Read the model definition and answer for the solid it produces. Units are mm, in the model's axes. A direction names the side the tool comes from. Coordinates: 2 decimals unless noted, no trailing zeros. Order: outer loops, then holes, each group sorted by start corner. A loop starts at its lowest first (then second) coordinate and runs counter-clockwise, first axis right, second up. Notation, with made-up numbers: (15, -25) -> (58, -25) arc R29 ccw to (58, 6) -> close; hole circle Ø5 at (79, 64.25). An arc over 180 degrees is marked (long way). Answer as a JSON object with one key per item and string values. Group by question number.
1) Section C-C on z = 34.5 is taken. Determine the outline of the cut face in (x, y) (3 decimals), and give its area (3 significant figures).
2) Section D-D on y = -20 is taken. Determine the outline of the cut face in (x, z) (3 decimals), and give its area (3 significant figures).
3) Section A-A on y = 0 is taken. Determine the outline of the cut face in (x, z) (3 decimals).
4) A tool of negligible diameter and unlimited length cuts with its end or side. For faces 1 (the cylindrical face through (30.18, 0.39, 66.19)), 2 (the flat face through (28.575, 0, 28)), from which of +Z, -Z, +X, -X, +Y, -Y can it reach the whole face along a straight path? Write none if from no direction.
5) Consider L1, parallel to Z at x = 30.8, y = 0; L2, parallel to X at y = -22, z = 9.5 (3 decimals); L3, parallel to Z at x = 25.5, y = -27 (3 decimals). Determine where each line is inside the solid, lowest interval first.
6) Determine the mould class of faces 3 (the cylindrical face through (30.18, -0.83, 59.79)), 4 (the flat face through (-31.75, 0, 25)), 5 (the flat face through (-28.575, 0, 28)), 6 (the flat face through (0, 0, 3.175)) for opening direction X: released by +X, released by -X, zero draft, split by the parting line, or undercut.
7) Given pin 1 (3 mm diameter, centred on x = -1, y = 7.5, fed in from -Z); pin 2 (8 mm diameter, centred on x = 24, z = 44.5, fed in from -Y); pin 3 (1 mm diameter, centred on x = -23.5, y = -5.5, fed in from +Z) (3 decimals), each flat-ended and moving along its own axis, determine where each tip first touches the part or whether it passes through.
8) Section B-B on z = 56 is taken. Determine the outline of the cut face in (x, y) (3 decimals).
from build123d import *

# Parameters (mm, degrees)
F0_W     = 31.75
F0_H     = 63.5
F1_DEPTH = 3.175
F2_R     = 6.35
F3_DEPTH = 3.175


with BuildPart() as f1:
    # F0 (on Top) → F1 (new body)
    with BuildSketch(Plane.XY):
        with Locations((15.875, 0)):
            Rectangle(F0_W, F0_H)
    extrude(amount=F1_DEPTH)

    # F2 (on face) → F3 (join)
    with BuildSketch(Plane.YZ.offset(31.75)):
        Polygon((-10.280992, 46.040436), (-30.269473, 3.175), (30.269473, 3.175), (10.280992, 46.040436), align=None)
        with BuildLine():
            ThreePointArc((10.280992, 46.040436), (0, 66.196386), (-10.280992, 46.040436))
            Line((-10.280992, 46.040436), (10.280992, 46.040436))
        make_face()
        with Locations((0, 53.496386)):
            Circle(F2_R, mode=Mode.SUBTRACT)
    extrude(amount=-F3_DEPTH)

    # F4: F1 across plane


with BuildPart() as f1_1:
    add(f1.part)
    add(f1.part.mirror(Plane.YZ))


solid = f1_1.part
Worked answers:
{
 "1": {"outline": "(-31.75, -15.662) -> (-28.575, -15.662) -> (-28.575, 15.662) -> (-31.75, 15.662) -> close; (28.575, -15.662) -> (31.75, -15.662) -> (31.75, 15.662) -> (28.575, 15.662) -> close", "area": "199 mm²"},
 "2": {"outline": "(-31.75, 0) -> (31.75, 0) -> (31.75, 25.198) -> (28.575, 25.198) -> (28.575, 3.175) -> (-28.575, 3.175) -> (-28.575, 25.198) -> (-31.75, 25.198) -> close", "area": "341 mm²"},
 "3": {"outline": "(-31.75, 0) -> (31.75, 0) -> (31.75, 47.146) -> (28.575, 47.146) -> (28.575, 3.175) -> (-28.575, 3.175) -> (-28.575, 47.146) -> (-31.75, 47.146) -> close; (-31.75, 59.846) -> (-28.575, 59.846) -> (-28.575, 66.196) -> (-31.75, 66.196) -> close; (28.575, 59.846) -> (31.75, 59.846) -> (31.75, 66.196) -> (28.575, 66.196) -> close"},
 "4": {"face 1": "+X, -X", "face 2": "+Z, +Y, -Y"},
 "5": {"L1": "z = 0 to 47.15, 59.85 to 66.2", "L2": "x = -31.75 to -28.575, 28.575 to 31.75", "L3": "z = 0 to 3.175"},
 "6": {"face 3": "zero draft", "face 4": "released by -X", "face 5": "undercut", "face 6": "undercut"},
 "7": {"pin 1": "stops at z = 0", "pin 2": "passes through", "pin 3": "stops at z = 3.175"},
 "8": {"outline": "(-31.75, -12.451) -> (-28.575, -12.451) -> (-28.575, -5.836) -> (-31.75, -5.836) -> close; (-31.75, 5.836) -> (-28.575, 5.836) -> (-28.575, 12.451) -> (-31.75, 12.451) -> close; (28.575, -12.451) -> (31.75, -12.451) -> (31.75, -5.836) -> (28.575, -5.836) -> close; (28.575, 5.836) -> (31.75, 5.836) -> (31.75, 12.451) -> (28.575, 12.451) -> close"}
}
